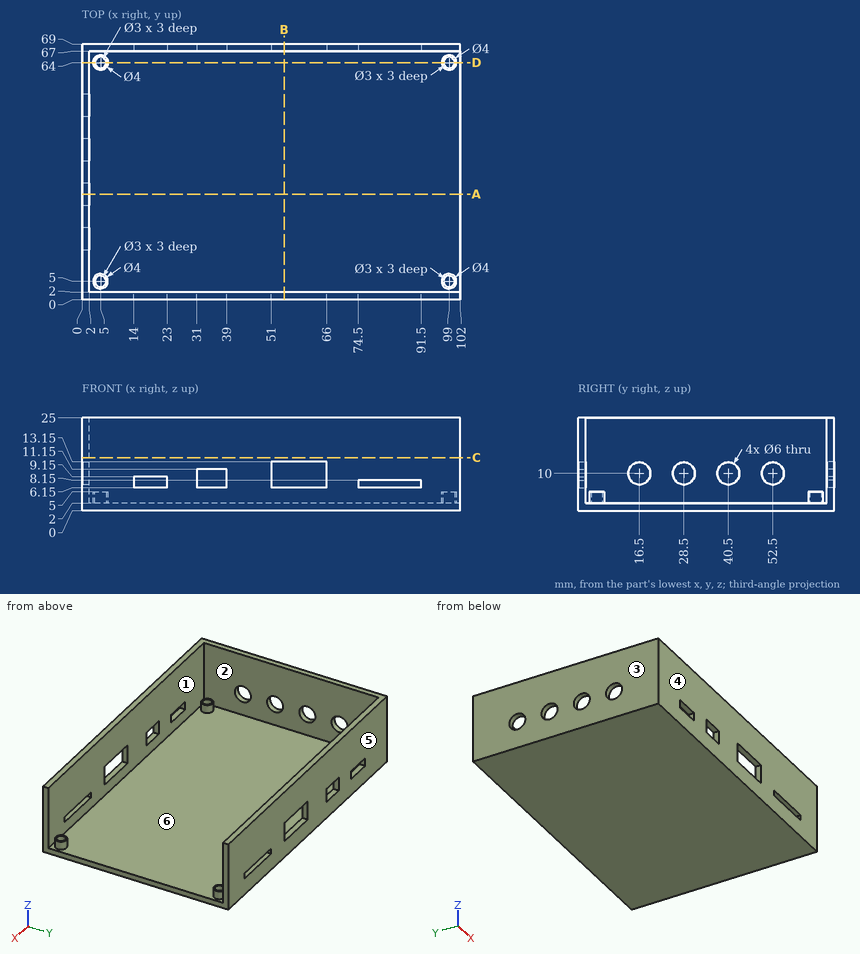
Verification items for this drawing (mm, ordinates from the low corner). A direction names the side the tool comes from. Round coordinates to 2 decimals unless told otherwise and drop trailing zeros. Order: outer loops, then holes, each group sorted by start corner. A loop starts at its lowest first (then second) coordinate and runs counter-clockwise, first axis right, second up. Notation, with made-up numbers: M 10.25,36 L 45.25,36 A11 ccw 45.25,55 Z; hole C -11,24 d6. An arc over 180 degrees is marked long. Answer in a Markdown table with one row per item. Add a question column.
Item 1: Sectioned sample at D-D, the plane y = 64. Enter the section's corners in (x, z).
Item 2: Sectioned sample at A-A, the plane y = 28.5. Enter the section's corners in (x, z), plus the area to 3 significant figures.
Item 3: Material ranges on L1, parallel to Y at x = 5, z = 2.8; L2, parallel to Y at x = 33, z = 17; L3, parallel to X at y = 5, z = 3.2, recorded low to high. Write a range as [from, to].
Item 4: Sectioned sample at C-C, the plane z = 14.25. Enter the section's corners in (x, y), plus the area to 3 significant figures.
Item 5: Sectioned sample at B-B, the plane x = 54.5. Enter the section's corners in (y, z).
Item 6: Depth check by flat-ended pin: pin 1 Ø2 at (y, z) = (0.5, 10) entering from -X; pin 2 Ø5 at (x, y) = (26, 22) entering from +Z; pin 3 Ø5 at (y, z) = (40.5, 10) entering from +X; pin 4 Ø3 at (x, y) = (99.5, 64.5) entering from +Z. Enter the tip coordinate at first touch or a pass-through.
Item 7: Set-up check for the marked faces 5 and 6: record each of +Z, -Z, +X, -X, +Y, -Y from which the full face is reachable in a straight line by a thin tool's end or side.
Item 8: Draft check along Y on the marked faces 1, 2, 3 and 4. Enter one of: released by +Y, released by -Y, zero draft, split by the parting line, or undercut.
Filled in:
| question | item | result |
|---|---|---|
| 1 | outline | M 0,0 L 102,0 L 102,2 L 101,2 L 101,5 L 100.5,5 L 100.5,2 L 97.5,2 L 97.5,5 L 97,5 L 97,2 L 7,2 L 7,5 L 6.5,5 L 6.5,2 L 3.5,2 L 3.5,5 L 3,5 L 3,2 L 2,2 L 2,25 L 0,25 Z |
| 2 | outline | M 0,0 L 102,0 L 102,2 L 2,2 L 2,7 L 0,7 Z; M 0,13 L 2,13 L 2,25 L 0,25 Z |
| 2 | area | 238 mm² |
| 3 | L1 | y = [0, 2], [3, 3.5], [6.5, 7], [62, 62.5], [65.5, 66], [67, 69] |
| 3 | L2 | y = [0, 2], [67, 69] |
| 3 | L3 | x = [0, 2], [3, 3.5], [6.5, 7], [97, 97.5], [100.5, 101] |
| 4 | outline | M 0,0 L 102,0 L 102,2 L 2,2 L 2,67 L 102,67 L 102,69 L 0,69 Z |
| 4 | area | 538 mm² |
| 5 | outline | M 0,0 L 69,0 L 69,6.15 L 67,6.15 L 67,2 L 2,2 L 2,6.15 L 0,6.15 Z; M 0,13.15 L 2,13.15 L 2,25 L 0,25 Z; M 67,13.15 L 69,13.15 L 69,25 L 67,25 Z |
| 6 | pin 1 | stops at x = 0 |
| 6 | pin 2 | stops at z = 2 |
| 6 | pin 3 | passes through |
| 6 | pin 4 | stops at z = 5 |
| 7 | face 5 | +Z, -Z, +X, -X, +Y |
| 7 | face 6 | +Z |
| 8 | face 1 | undercut |
| 8 | face 2 | undercut |
| 8 | face 3 | zero draft |
| 8 | face 4 | released by -Y |
